Could you check a few things on this model? Use its own coordinates, in mm. A direction names the side the tool comes from. Round coordinates to 2 decimals unless told otherwise and drop trailing zeros. Order: outer loops, then holes, each group sorted by start corner. A loop starts at its lowest first (then second) coordinate and runs counter-clockwise, first axis right, second up. Notation, with made-up numbers: (11, -26.5) - (44, -26.5) arc R10 cw to (44, -20.5) - close; hole circle Ø6 at (83, 20). An arc over 180 degrees is marked (long way). Use one line per item in the form item = value.
from build123d import *
from build123d import SkipClean  # not in build123d's __all__

# Parameters (mm, degrees)
F1_DEPTH  = 103.9495
F3_R      = 12.7
F4_DEPTH  = 19.05
F6_DEPTH  = 25.4
F8_DEPTH  = 2.54
F9_R      = 12.7
F10_DEPTH = 52.451


# Not quite as in the source:
# - after a boolean that leaves OpenCascade's solid faulty, fix() repairs it


with BuildPart() as f1:
    # F0 (on Right) → F1 (new body, symmetric)
    with BuildSketch(Plane.YZ):
        with BuildLine():
            ThreePointArc((12.4434078933, -2.54), (12.6356891432, -1.2764638175), (12.7, 0))
            ThreePointArc((12.7, 0), (12.6356891432, 1.2764638175), (12.4434078933, 2.54))
            Line((12.4434078933, 2.54), (5.8198711326, 2.54))
            ThreePointArc((5.8198711326, 2.54), (6.2160550871, 1.2973662374), (6.35, 0))
            ThreePointArc((6.35, 0), (6.2160550871, -1.2973662374), (5.8198711326, -2.54))
            Line((5.8198711326, -2.54), (12.4434078933, -2.54))
        make_face()
        with BuildLine():
            Line((5.8198711326, 2.54), (12.4434078933, 2.54))
            ThreePointArc((12.4434078933, 2.54), (8.9802561211, 8.9802561211), (2.54, 12.4434078933))
            Line((2.54, 12.4434078933), (2.54, 5.8198711326))
            ThreePointArc((2.54, 5.8198711326), (4.4901280605, 4.4901280605), (5.8198711326, 2.54))
        make_face()
        with BuildLine():
            ThreePointArc((2.54, -12.4434078933), (8.9802561211, -8.9802561211), (12.4434078933, -2.54))
            Line((12.4434078933, -2.54), (5.8198711326, -2.54))
            ThreePointArc((5.8198711326, -2.54), (4.4901280605, -4.4901280605), (2.54, -5.8198711326))
            Line((2.54, -5.8198711326), (2.54, -12.4434078933))
        make_face()
        with BuildLine():
            Line((2.54, 5.8198711326), (2.54, 12.4434078933))
            ThreePointArc((2.54, 12.4434078933), (0, 12.7), (-2.54, 12.4434078933))
            Line((-2.54, 12.4434078933), (-2.54, 5.8198711326))
            ThreePointArc((-2.54, 5.8198711326), (0, 6.35), (2.54, 5.8198711326))
        make_face()
        with BuildLine():
            ThreePointArc((-2.54, -12.4434078933), (0, -12.7), (2.54, -12.4434078933))
            Line((2.54, -12.4434078933), (2.54, -5.8198711326))
            ThreePointArc((2.54, -5.8198711326), (0, -6.35), (-2.54, -5.8198711326))
            Line((-2.54, -5.8198711326), (-2.54, -12.4434078933))
        make_face()
        with BuildLine():
            Line((-2.54, 5.8198711326), (-2.54, 12.4434078933))
            ThreePointArc((-2.54, 12.4434078933), (-8.9802561211, 8.9802561211), (-12.4434078933, 2.54))
            Line((-12.4434078933, 2.54), (-5.8198711326, 2.54))
            ThreePointArc((-5.8198711326, 2.54), (-4.4901280605, 4.4901280605), (-2.54, 5.8198711326))
        make_face()
        with BuildLine():
            ThreePointArc((-12.4434078933, -2.54), (-8.9802561211, -8.9802561211), (-2.54, -12.4434078933))
            Line((-2.54, -12.4434078933), (-2.54, -5.8198711326))
            ThreePointArc((-2.54, -5.8198711326), (-4.4901280605, -4.4901280605), (-5.8198711326, -2.54))
            Line((-5.8198711326, -2.54), (-12.4434078933, -2.54))
        make_face()
        with BuildLine():
            Line((-5.8198711326, 2.54), (-12.4434078933, 2.54))
            ThreePointArc((-12.4434078933, 2.54), (-12.7, 0), (-12.4434078933, -2.54))
            Line((-12.4434078933, -2.54), (-5.8198711326, -2.54))
            ThreePointArc((-5.8198711326, -2.54), (-6.35, 0), (-5.8198711326, 2.54))
        make_face()
        with BuildLine():
            ThreePointArc((6.35, 0), (6.2160550871, 1.2973662374), (5.8198711326, 2.54))
            ThreePointArc((5.8198711326, 2.54), (4.4901280605, 4.4901280605), (2.54, 5.8198711326))
            ThreePointArc((2.54, 5.8198711326), (0, 6.35), (-2.54, 5.8198711326))
            ThreePointArc((-2.54, 5.8198711326), (-4.4901280605, 4.4901280605), (-5.8198711326, 2.54))
            ThreePointArc((-5.8198711326, 2.54), (-6.35, 0), (-5.8198711326, -2.54))
            ThreePointArc((-5.8198711326, -2.54), (-4.4901280605, -4.4901280605), (-2.54, -5.8198711326))
            ThreePointArc((-2.54, -5.8198711326), (0, -6.35), (2.54, -5.8198711326))
            ThreePointArc((2.54, -5.8198711326), (4.4901280605, -4.4901280605), (5.8198711326, -2.54))
            ThreePointArc((5.8198711326, -2.54), (6.2160550871, -1.2973662374), (6.35, 0))
        make_face()
    extrude(amount=F1_DEPTH, both=True)

    # F3 (on face) → F4 (join)
    with BuildSketch(Plane.YZ.offset(103.9495)):
        Circle(F3_R)
    with SkipClean():  # cleaning this boolean's faces spoils the solid; the shape is the same uncleaned
        extrude(amount=F4_DEPTH)

    # F5 (on face) → F6 (cut)
    with BuildSketch(Plane.YZ.offset(122.9995)):
        with BuildLine():
            ThreePointArc((5.8198711326, -2.54), (6.2160550871, -1.2973662374), (6.35, 0))
            ThreePointArc((6.35, 0), (6.2160550871, 1.2973662374), (5.8198711326, 2.54))
            ThreePointArc((5.8198711326, 2.54), (4.4901280605, 4.4901280605), (2.54, 5.8198711326))
            ThreePointArc((2.54, 5.8198711326), (0, 6.35), (-2.54, 5.8198711326))
            ThreePointArc((-2.54, 5.8198711326), (-4.4901280605, 4.4901280605), (-5.8198711326, 2.54))
            ThreePointArc((-5.8198711326, 2.54), (-6.35, 0), (-5.8198711326, -2.54))
            ThreePointArc((-5.8198711326, -2.54), (-4.4901280605, -4.4901280605), (-2.54, -5.8198711326))
            ThreePointArc((-2.54, -5.8198711326), (0, -6.35), (2.54, -5.8198711326))
            ThreePointArc((2.54, -5.8198711326), (4.4901280605, -4.4901280605), (5.8198711326, -2.54))
        make_face()
    extrude(amount=-F6_DEPTH, mode=Mode.SUBTRACT)

    add(f1.part.fix(), mode=Mode.REPLACE)

    # F7 (on face) → F8 (cut)
    with BuildSketch(Plane.YZ.offset(122.9995)):
        with BuildLine():
            ThreePointArc((2.54, 12.4434078933), (0, 12.7), (-2.54, 12.4434078933))
            Line((-2.54, 12.4434078933), (-2.54, 5.8198711326))
            ThreePointArc((-2.54, 5.8198711326), (0, 6.35), (2.54, 5.8198711326))
            Line((2.54, 5.8198711326), (2.54, 12.4434078933))
        make_face()
        with BuildLine():
            ThreePointArc((12.7, 0), (12.6356891432, 1.2764638175), (12.4434078933, 2.54))
            Line((12.4434078933, 2.54), (5.8198711326, 2.54))
            ThreePointArc((5.8198711326, 2.54), (6.2160550871, 1.2973662374), (6.35, 0))
            ThreePointArc((6.35, 0), (6.2160550871, -1.2973662374), (5.8198711326, -2.54))
            Line((5.8198711326, -2.54), (12.4434078933, -2.54))
            ThreePointArc((12.4434078933, -2.54), (12.6356891432, -1.2764638175), (12.7, 0))
        make_face()
        with BuildLine():
            Line((-2.54, -5.8198711326), (-2.54, -12.4434078933))
            ThreePointArc((-2.54, -12.4434078933), (0, -12.7), (2.54, -12.4434078933))
            Line((2.54, -12.4434078933), (2.54, -5.8198711326))
            ThreePointArc((2.54, -5.8198711326), (0, -6.35), (-2.54, -5.8198711326))
        make_face()
        with BuildLine():
            Line((-5.8198711326, 2.54), (-12.4434078933, 2.54))
            ThreePointArc((-12.4434078933, 2.54), (-12.7, 0), (-12.4434078933, -2.54))
            Line((-12.4434078933, -2.54), (-5.8198711326, -2.54))
            ThreePointArc((-5.8198711326, -2.54), (-6.35, 0), (-5.8198711326, 2.54))
        make_face()
    extrude(amount=-F8_DEPTH, mode=Mode.SUBTRACT)

    # F9 (on face) → F10 (join)
    with BuildSketch(Plane(origin=(-103.9495, 0, 0), x_dir=(0, -1, 0), z_dir=(-1, 0, 0))):
        Circle(F9_R)
    with SkipClean():  # cleaning this boolean's faces spoils the solid; the shape is the same uncleaned
        extrude(amount=F10_DEPTH)


solid = f1.part
Item 1: Imagine slicing it at A-A on y = 0. Please give me the cut outline in (x, z), plus the area to 3 significant figures.
Found:
outline = (-156.4, -12.7) - (120.46, -12.7) - (120.46, -6.35) - (97.6, -6.35) - (97.6, 6.35) - (120.46, 6.35) - (120.46, 12.7) - (-156.4, 12.7) - close
area = 6,740 mm2
Item 2: Imagine slicing it at C-C on z = 9.5. Please give me the cut outline in (x, y).
Found:
outline = (-156.4, -8.43) - (123, -8.43) - (123, -2.54) - (120.46, -2.54) - (120.46, 2.54) - (123, 2.54) - (123, 8.43) - (-156.4, 8.43) - close
Item 3: I need wall thicknesses on L1, parallel to Y at x = 78, z = 2.25; L2, parallel to Z at x = 99.5, y = -4; L3, parallel to X at y = 0.5, z = 5.75. Which ranges of each line are inside material? Lowest first, please.
Found:
L1 = -12.5 to 12.5
L2 = -12.05 to -4.93, 4.93 to 12.05
L3 = -156.4 to 97.6
Item 4: If we mould it in two halves opening along Y, with no side actions, what happens to faces 4 (the face through (-156.4, 0, 0)), 5 (the face through (97.6, 0, 0))? For each: released by +Y, released by -Y, zero draft, split by the parting line, or undercut.
Found:
face_4 = zero draft
face_5 = undercut
Item 5: Imagine slicing it at B-B on x = -140. Please give me the cut outline in (y, z).
Found:
outline = circle Ø25.4 at (0, 0)
Item 6: For faces 1 (the face through (123, 6, -6)), 2 (the face through (120.459, 0, 9)), 3 (the face through (120.459, -9, 0)), which set-ups out of +Z, -Z, +X, -X, +Y, -Y let a thin tool reach every point of the face, with its end or its side?
Found:
face_1 = +Z, -Z, +X, +Y, -Y
face_2 = +Z, -Z, +X
face_3 = +X, +Y, -Y
Item 7: Will these pins go through, and if not, where does the flat tip stop? P1, Ø1.5, axis at y = -0.5, z = -10.5, coming from the +X side; P2, Ø0.8, axis at x = 122, z = 7.5, coming from the -Y side; P3, Ø2, axis at x = 122.5, z = -10, coming from the -Y side.
Found:
P1 = 120.46
P2 = -10.53
P3 = -8.96
